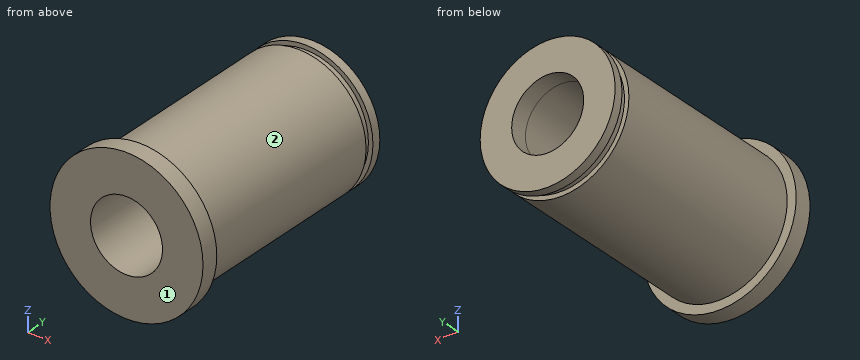
```python
from build123d import *

# Parameters (mm, degrees)
F0_R     = 8.5
F0_R_2   = 7.5
F0_R_3   = 7
F0_R_4   = 4
F1_DEPTH = 25
F2_DEPTH = 23
F3_DEPTH = 2
F4_DEPTH = 1


with BuildPart() as f1:
    # F0 (on Front) → F1 (new body)
    with BuildSketch(Plane.XZ):
        Circle(F0_R)
        Circle(F0_R_2, mode=Mode.SUBTRACT)
        Circle(F0_R_2)
        Circle(F0_R_3, mode=Mode.SUBTRACT)
        Circle(F0_R_3)
        Circle(F0_R_4, mode=Mode.SUBTRACT)
    extrude(amount=F1_DEPTH)

    # F0 (on Front) → F2 (cut)
    with BuildSketch(Plane.XZ):
        Circle(F0_R)
        Circle(F0_R_2, mode=Mode.SUBTRACT)
    extrude(amount=F2_DEPTH, mode=Mode.SUBTRACT)

    # F0 (on Front) → F3 (join)
    with BuildSketch(Plane.XZ):
        Circle(F0_R_2)
        Circle(F0_R_3, mode=Mode.SUBTRACT)
        Circle(F0_R_3)
        Circle(F0_R_4, mode=Mode.SUBTRACT)
    extrude(amount=-F3_DEPTH)

    # F0 (on Front) → F4 (cut)
    with BuildSketch(Plane.XZ):
        Circle(F0_R_2)
        Circle(F0_R_3, mode=Mode.SUBTRACT)
    extrude(amount=-F4_DEPTH, mode=Mode.SUBTRACT)


solid = f1.part
```
Geometry: final body of the model. Coordinates: model frame, mm. Face numbers are marked on the shaded views. Coordinates: 2 decimals unless noted, no trailing zeros. Order: outer loops, then holes, each group sorted by start corner. A loop starts at its lowest first (then second) coordinate and runs counter-clockwise, first axis right, second up. Notation, with made-up numbers: M 67.5,47 L 93.5,47 A20 ccw 93.5,71 Z; hole C 82.25,18 d5. An arc over 180 degrees is marked long. Answer in a Markdown table with one row per item. Add a question column.
Q1. Line query: L1, parallel to Z at x = 0, y = 1.1; L2, parallel to Y at x = 7.25, z = -4.25; L3, parallel to Z at x = 3.25, y = -8.5. Output: solid intervals per line, ascending.
Q2. Contact query for flat-ended pins moving along their axis: P1, Ø7, axis at x = 0, z = 0, coming from the -Y side; P2, Ø5, axis at x = -2.5, y = -1.5, coming from the -Z side; P3, Ø4.5, axis at x = -1, z = -3.5, coming from the -Y side; P4, Ø3, axis at y = -4.5, z = -1.5, coming from the -X side. Output: stop coordinate, or through.
Q3. Section query B-B on z = 0. Return the cut outline in (x, y).
Q4. Section query A-A on x = 0. Return the cut outline in (y, z), and give its area (3 significant figures).
Q5. Mould query, pull axis Z, two halves, no side actions, for the marked faces 1 and 2. Classes: released by +Z, released by -Z, zero draft, split by the parting line, or undercut.
Q6. Section query D-D on x = -6.25. Return the cut outline in (y, z).
Q7. Section query C-C on y = -21. Return the cut outline in (x, z), and give its area (3 significant figures).
Completed:
| question | item | result |
|---|---|---|
| 1 | L1 | z = -7.5 to -4, 4 to 7.5 |
| 1 | L2 | y = -25 to -23 |
| 1 | L3 | z = -6.76 to -2.33, 2.33 to 6.76 |
| 2 | P1 | passes through |
| 2 | P2 | stops at z = -7.5 |
| 2 | P3 | stops at y = -25 |
| 2 | P4 | stops at x = -7.5 |
| 3 | outline | M -8.5,-25 L -4,-25 L -4,2 L -7.5,2 L -7.5,1 L -7,1 L -7,0 L -7.5,0 L -7.5,-23 L -8.5,-23 Z; M 4,-25 L 8.5,-25 L 8.5,-23 L 7.5,-23 L 7.5,0 L 7,0 L 7,1 L 7.5,1 L 7.5,2 L 4,2 Z |
| 4 | outline | M -25,-8.5 L -23,-8.5 L -23,-7.5 L 0,-7.5 L 0,-7 L 1,-7 L 1,-7.5 L 2,-7.5 L 2,-4 L -25,-4 Z; M -25,4 L 2,4 L 2,7.5 L 1,7.5 L 1,7 L 0,7 L 0,7.5 L -23,7.5 L -23,8.5 L -25,8.5 Z |
| 4 | area | 192 mm2 |
| 5 | face 1 | zero draft |
| 5 | face 2 | split by the parting line |
| 6 | outline | M -25,-5.76 L -23,-5.76 L -23,-4.15 L 0,-4.15 L 0,-3.15 L 1,-3.15 L 1,-4.15 L 2,-4.15 L 2,4.15 L 1,4.15 L 1,3.15 L 0,3.15 L 0,4.15 L -23,4.15 L -23,5.76 L -25,5.76 Z |
| 7 | outline | C 0,0 d15; hole C 0,0 d8 |
| 7 | area | 126 mm2 |
